The model under review builds one solid part; all positions refer to its coordinate system, in mm. Give positions to 0.01 mm unless a question says otherwise; leave off trailing zeros. Write each loop counter-clockwise with the first axis right and the second up, starting at its lowest first coordinate (ties: lowest second). Pieces come first, ordered by that corner, then holes. Notation, with made-up numbers: (17.5, -11) -> (62.5, -11) arc R21 cw to (62.5, 8) -> close; hole circle Ø10 at (88.25, 59). An arc over 180 degrees is marked (long way). Use CSV: the item, a comma, the result in double quotes.
```python
from build123d import *

# Parameters (mm, degrees)
F0_W     = 540
F0_H     = 390
F1_DEPTH = 10
F2_W     = 80
F2_H     = 80
F2_R     = 15
F3_DEPTH = 10


with BuildPart() as f1:
    # F0 (on Front) → F1 (new body)
    with BuildSketch(Plane.XZ):
        Polygon((-575.5810141563, 243.9473703504), (-465.5810141563, -206.0526296496), (133.660423523, -206.0526296496), (243.660423523, 243.9473703504), (133.660423523, 243.9473703504), (-465.5810141563, 243.9473703504), align=None)
        with Locations((-166.339576477, 18.9473703504)):
            Rectangle(F0_W, F0_H, mode=Mode.SUBTRACT)
        Polygon((-495.5810141563, 43.0153865893), (-537.3643879646, 213.9473703504), (-495.5810141563, 213.9473703504), align=None, mode=Mode.SUBTRACT)
        Polygon((163.660423523, 213.9473703504), (205.4437973313, 213.9473703504), (163.660423523, 43.0153865893), align=None, mode=Mode.SUBTRACT)
    extrude(amount=F1_DEPTH)

    # F2 (on face) → F3 (join)
    with BuildSketch(Plane.XZ.offset(10)):
        with Locations((-396.339576477, 173.9473703504)):
            Rectangle(F2_W, F2_H)
        with Locations((-396.339576477, 198.8157841563)):
            Circle(F2_R, mode=Mode.SUBTRACT)
        with Locations((63.660423523, 173.9473703504)):
            Rectangle(F2_W, F2_H)
        with Locations((63.660423523, 198.8157841563)):
            Circle(F2_R, mode=Mode.SUBTRACT)
        with Locations((63.660423523, -136.0526296496)):
            Rectangle(F2_W, F2_H)
        with Locations((63.660423523, -136.0526296496)):
            Circle(F2_R, mode=Mode.SUBTRACT)
        with Locations((-396.339576477, -136.0526296496)):
            Rectangle(F2_W, F2_H)
        with Locations((-396.339576477, -136.0526296496)):
            Circle(F2_R, mode=Mode.SUBTRACT)
    extrude(amount=-F3_DEPTH)


solid = f1.part
```
Q1. Consider section B-B (z = -46.5). Write out the cut boundary in (x, y).
Derived:
outline,"(-504.58, -10) -> (-436.34, -10) -> (-436.34, 0) -> (-504.58, 0) -> close; (103.66, -10) -> (172.66, -10) -> (172.66, 0) -> (103.66, 0) -> close"
Q2. To check wall thickness, follow probe 1 along X at (y, z) = (-7.5, 115); probe 2 along Z at (x, y) = (-103, -4.5); probe 3 along Z at (x, y) = (71, -4). State the ranges of each line that lie inside material, in increasing order.
Derived:
probe 1,"x = -544.06 to -513.18, -495.58 to -436.34, 103.66 to 163.66, 181.26 to 212.14"
probe 2,"z = -206.05 to -176.05, 213.95 to 243.95"
probe 3,"z = -206.05 to -149.13, -122.97 to -96.05, 133.95 to 185.73, 211.9 to 243.95"
Q3. Consider section A-A (x = -94.5). Write out the cut boundary in (y, z), then the cut area to 3 significant figures.
Derived:
outline,"(-10, -206.05) -> (0, -206.05) -> (0, -176.05) -> (-10, -176.05) -> close; (-10, 213.95) -> (0, 213.95) -> (0, 243.95) -> (-10, 243.95) -> close"
area,"600 mm2"
Q4. Insertion check: pin 1 (1 mm diameter, centred on y = -6.5, z = -91, fed in from -X); pin 2 (3 mm diameter, centred on y = -8, z = 142.5, fed in from -X); pin 3 (3 mm diameter, centred on y = -6.5, z = 189, fed in from +X). Each pin has a flat end and moves straight along its axis. Give the tip position at first contact, or say it passes through.
Derived:
pin 1,"stops at x = -493.83"
pin 2,"stops at x = -551.15"
pin 3,"stops at x = 230.6"
Q5. The part is to be moulded in two halves that separate along X. For faces 1 (the flat face through (184.845, -4.93, 129.678)), 2 (the flat face through (187.89, -4.93, 15.8)), 3 (the flat face through (-138, 0, 220)), say which applies: pulls with the +X half, pulls with the -X half, needs draft (parallel to the pull), parting line crosses it, or undercut.
Derived:
face 1,"undercut"
face 2,"pulls with the +X half"
face 3,"needs draft"
Q6. Consider section D-D (z = 73). Write out the cut boundary in (x, y).
Derived:
outline,"(-533.79, -10) -> (-502.91, -10) -> (-502.91, 0) -> (-533.79, 0) -> close; (-495.58, -10) -> (-436.34, -10) -> (-436.34, 0) -> (-495.58, 0) -> close; (103.66, -10) -> (163.66, -10) -> (163.66, 0) -> (103.66, 0) -> close; (170.99, -10) -> (201.87, -10) -> (201.87, 0) -> (170.99, 0) -> close"
Q7. Consider section C-C (x = 57). Write out the cut boundary in (y, z).
Derived:
outline,"(-10, -206.05) -> (0, -206.05) -> (0, -149.49) -> (-10, -149.49) -> close; (-10, -122.61) -> (0, -122.61) -> (0, -96.05) -> (-10, -96.05) -> close; (-10, 133.95) -> (0, 133.95) -> (0, 185.38) -> (-10, 185.38) -> close; (-10, 212.26) -> (0, 212.26) -> (0, 243.95) -> (-10, 243.95) -> close"
